from build123d import *

# Parameters (mm, degrees)
T_LE_DE_BASE_PLI_E1_DEPTH             = 20.5
ESQUISSE8_W                           = 24
ESQUISSE8_H                           = 2
BOSS_EXTRU_1_DEPTH                    = 8.5
T_LE_PLI_E_SUR_AR_TE1_STRIP_W         = 10
T_LE_PLI_E_SUR_AR_TE1_STRIP_H         = 2
T_LE_PLI_E_SUR_AR_TE1_STRIP_CUT_DEPTH = 8.5
T_LE_PLI_E_SUR_AR_TE1_DEPTH           = 8.5
ESQUISSE12_W                          = 1.5
ESQUISSE12_H                          = 12
ENL_V_MAT_EXTRU_1_DEPTH               = 8.5
DIAM_TRE_DU_PER_AGE_4_0_4_1_D         = 4
DIAM_TRE_DU_PER_AGE_8_0_8_1_D         = 8
DIAM_TRE_DU_PER_AGE_2_5_2_5_1_D       = 2.5
R_P_TITION_CIRCULAIRE1_COUNT          = 8
DIAM_TRE_DU_PER_AGE_4_0_4_2_D         = 4
DIAM_TRE_DU_PER_AGE_2_5_2_5_2_D       = 2.5
CONG_1_R                              = 4
DIAM_TRE_DU_PER_AGE_8_0_8_2_D         = 8
DIAM_TRE_DU_PER_AGE_2_5_2_5_3_D       = 2.5
R_P_TITION_CIRCULAIRE2_COUNT          = 4
CROQUIS1_R                            = 2.5
CORTAR_EXTRUIR1_DEPTH                 = 10


# Sheet-metal steps are written as plain solids
with BuildPart() as part:
    # Esquisse1 → Tôle de base pliée1 (new body)
    with BuildSketch(Plane(origin=(0, 0, 0), x_dir=(0, 0, -1), z_dir=(1, 0, 0))):
        with BuildLine():
            Line((0, 27), (0, 3))
            ThreePointArc((0, 3), (-0.878679656, 0.878679656), (-3, 0))
            Line((-3, 0), (-37.5, 0))
            Line((-37.5, 0), (-37.5, 2))
            Line((-37.5, 2), (-3, 2))
            ThreePointArc((-3, 2), (-2.292893219, 2.292893219), (-2, 3))
            Line((-2, 3), (-2, 27))
            Line((-2, 27), (0, 27))
        make_face()
    extrude(amount=T_LE_DE_BASE_PLI_E1_DEPTH)

    # Esquisse8 → Boss.-Extru.1 (add)
    with BuildSketch(Plane(origin=(20.5, 0, 0), x_dir=(0, 0, -1), z_dir=(1, 0, 0))):
        with Locations((-19, 1)):
            Rectangle(ESQUISSE8_W, ESQUISSE8_H)
    extrude(amount=BOSS_EXTRU_1_DEPTH)

    # Tôle pliée sur arête1 strip (across the edge) → Tôle pliée sur arête1 strip cut (cut)
    with BuildSketch(Plane(origin=(20.5, 2, 31), x_dir=(0, 0, -1), z_dir=(1, 0, 0))):
        with Locations((-4, -1)):
            Rectangle(T_LE_PLI_E_SUR_AR_TE1_STRIP_W, T_LE_PLI_E_SUR_AR_TE1_STRIP_H)
    extrude(amount=T_LE_PLI_E_SUR_AR_TE1_STRIP_CUT_DEPTH, mode=Mode.SUBTRACT)

    # Tôle pliée sur arête1 section (across the edge) → Tôle pliée sur arête1 (add)
    with BuildSketch(Plane(origin=(20.5, 2, 31), x_dir=(0, 0, -1), z_dir=(1, 0, 0))):
        with BuildLine():
            Line((-2, 1), (-2, 25))
            Line((-2, 25), (0, 25))
            Line((0, 25), (0, 1))
            ThreePointArc((0, 1), (0.292893219, 0.292893219), (1, 0))
            Line((1, 0), (1, -2))
            ThreePointArc((1, -2), (-1.121320344, -1.121320344), (-2, 1))
        make_face()
    extrude(amount=T_LE_PLI_E_SUR_AR_TE1_DEPTH)

    # Esquisse12 → Enlèv. mat.-Extru.1 (cut)
    with BuildSketch(Plane(origin=(0, 2, 0), x_dir=(1, 0, 0), z_dir=(0, 1, 0))):
        with Locations((19.75, -31.5)):
            Rectangle(ESQUISSE12_W, ESQUISSE12_H)
    extrude(amount=-ENL_V_MAT_EXTRU_1_DEPTH, mode=Mode.SUBTRACT)

    # Diamètre du perçage Ø4.0 (4)1 (through all)
    with Locations(Plane(origin=(0, 2, 0), x_dir=(1, 0, 0), z_dir=(0, 1, 0))):
        with Locations((24.25, -12.13), (24.25, -22.13)):
            Hole(DIAM_TRE_DU_PER_AGE_4_0_4_1_D / 2)

    # Diamètre du perçage Ø8.0 (8)1 (through all)
    with Locations(Plane(origin=(0, 2, 0), x_dir=(1, 0, 0), z_dir=(0, 1, 0))):
        with Locations((9.75, -25.5)):
            Hole(DIAM_TRE_DU_PER_AGE_8_0_8_1_D / 2)

    # Diamètre du perçage Ø2.5 (2.5)1 (through all)
    with Locations(Plane(origin=(0, 2, 0), x_dir=(1, 0, 0), z_dir=(0, 1, 0))):
        with Locations((9.75, -18.5)):
            diam_tre_du_per_age_2_5_2_5_1 = Hole(DIAM_TRE_DU_PER_AGE_2_5_2_5_1_D / 2)

    # Répétition circulaire1: Diamètre du perçage Ø2.5 (2.5)1 ×8 about axis, 3 skipped
    r_p_tition_circulaire1_axis = Axis((9.75, 2, 25.5), (0, 1, 0))
    add([diam_tre_du_per_age_2_5_2_5_1.rotate(r_p_tition_circulaire1_axis, i * 360 / R_P_TITION_CIRCULAIRE1_COUNT) for i in range(1, R_P_TITION_CIRCULAIRE1_COUNT) if i not in (1, 3, 6)], mode=Mode.SUBTRACT)

    # Diamètre du perçage Ø4.0 (4)2 (through all)
    with Locations(Plane.XY.offset(33)):
        with Locations((24.25, 19.87), (24.25, 9.87)):
            Hole(DIAM_TRE_DU_PER_AGE_4_0_4_2_D / 2)

    # Diamètre du perçage Ø2.5 (2.5)2 (through all)
    with Locations(Plane.XY.offset(2)):
        with Locations((10, 14.87)):
            Hole(DIAM_TRE_DU_PER_AGE_2_5_2_5_2_D / 2)

    # Congé1
    cong_1_edges = [part.edges().sort_by_distance(p)[0] for p in [
        (20.5, 27, 1),
        (29, 1, 7),
        (29, 27, 32),
        (19, 1, 37.5),
    ]]
    fillet(cong_1_edges, radius=CONG_1_R)

    # Symétrie1: part across plane


with BuildPart() as part_1:
    add(part.part)
    add(part.part.mirror(Plane(origin=(0, 3, 3), x_dir=(0, 0, 1), z_dir=(1, 0, 0))))

    # Diamètre du perçage Ø8.0 (8)2 (through all)
    with Locations(Plane(origin=(0, 2, 0), x_dir=(1, 0, 0), z_dir=(0, 1, 0))):
        with Locations((0, -12.13)):
            Hole(DIAM_TRE_DU_PER_AGE_8_0_8_2_D / 2)

    # Diamètre du perçage Ø2.5 (2.5)3 (through all)
    with Locations(Plane(origin=(0, 2, 0), x_dir=(1, 0, 0), z_dir=(0, 1, 0))):
        with Locations((0, -5.13)):
            diam_tre_du_per_age_2_5_2_5_3 = Hole(DIAM_TRE_DU_PER_AGE_2_5_2_5_3_D / 2)

    # Répétition circulaire2: Diamètre du perçage Ø2.5 (2.5)3 ×4 about axis
    r_p_tition_circulaire2_axis = Axis((0, 0, 12.13), (0, 1, 0))
    for i in range(1, R_P_TITION_CIRCULAIRE2_COUNT):
        add(diam_tre_du_per_age_2_5_2_5_3.rotate(r_p_tition_circulaire2_axis, i * 360 / R_P_TITION_CIRCULAIRE2_COUNT), mode=Mode.SUBTRACT)

    # Croquis1 → Cortar-Extruir1 (cut)
    with BuildSketch(Plane.XY.offset(2)):
        with Locations((10, 14.87)):
            Circle(CROQUIS1_R)
        with Locations((-10, 14.87)):
            Circle(CROQUIS1_R)
    extrude(amount=-CORTAR_EXTRUIR1_DEPTH, mode=Mode.SUBTRACT)


solid = part_1.part
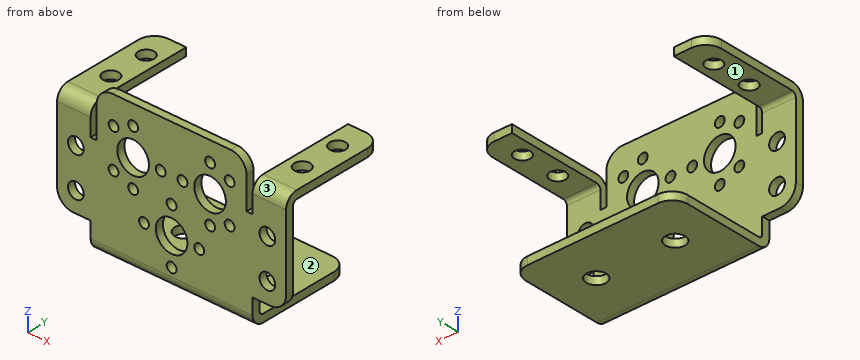
For this review, take the finished solid that the model builds, in its own axes (mm). Face numbers are marked on the shaded views. A direction names the side the tool comes from. Round coordinates to 2 decimals unless told otherwise and drop trailing zeros. Write each loop counter-clockwise with the first axis right and the second up, starting at its lowest first coordinate (ties: lowest second). Pieces come first, ordered by that corner, then holes. Notation, with made-up numbers: (25.25, 11) - (58.25, 11) arc R12 cw to (58.25, 31) - close; hole circle Ø10 at (19, -9.75). An arc over 180 degrees is marked (long way). Use a Markdown table: item, result.
Q1. We need section B-B (y = 14.87). Give the boundary of the cut face in (x, z), plus the area to 3 significant figures.
Derived:
| item | result |
|---|---|
| outline | (-29, 31) - (-20.5, 31) - (-20.5, 33) - (-29, 33) - close; (-20.5, 0) - (-12.5, 0) - (-12.5, 2) - (-20.5, 2) - close; (-7.5, 0) - (7.5, 0) - (7.5, 2) - (-7.5, 2) - close; (12.5, 0) - (20.5, 0) - (20.5, 2) - (12.5, 2) - close; (20.5, 31) - (29, 31) - (29, 33) - (20.5, 33) - close |
| area | 96.0 mm2 |
Q2. We need section D-D (x = -10). Give the boundary of the cut face in (y, z), plus the area to 3 significant figures.
Derived:
| item | result |
|---|---|
| outline | (0, 3) arc R3 ccw to (3, 0) - (12.37, 0) - (12.37, 2) - (3, 2) arc R1 cw to (2, 3) - (2, 17.28) - (0, 17.28) - close; (0, 19.72) - (2, 19.72) - (2, 21.51) - (0, 21.51) - close; (0, 29.49) - (2, 29.49) - (2, 31.28) - (0, 31.28) - close; (0, 33.72) - (2, 33.72) - (2, 37.5) - (0, 37.5) - close; (17.37, 0) - (27, 0) - (27, 2) - (17.37, 2) - close |
| area | 87.5 mm2 |
Q3. Wall thickness on line 1 along X through (y, z) = (0.8, 22.13); line 2 along Z through (x, y) = (-9.75, 1.1); line 3 along X through (y, z) = (1.3, 18.5): over which ranges is each line inside the solid? List them lowest first.
Derived:
| item | result |
|---|---|
| line 1 | x = -29 to -26.25, -22.25 to -11.9, -7.6 to 7.6, 11.9 to 22.25, 26.25 to 29 |
| line 2 | z = 0.68 to 17.25, 19.75 to 21.5, 29.5 to 31.25, 33.75 to 37.5 |
| line 3 | x = -29 to -11, -8.5 to -1.08, 1.08 to 8.5, 11 to 29 |
Q4. Machinability: for the marked faces 1, 2 and 3, which of the approach directions +Z, -Z, +X, -X, +Y, -Y give a long, thin tool a straight path to every point of the face, cutting with its end or side? Answer none if there is none.
Derived:
| item | result |
|---|---|
| face 1 | -Z, +X, -X, +Y |
| face 2 | +Z, +X, -X, +Y |
| face 3 | +Z, +X, -Y |
Q5. We need section A-A (x = 0). Give the boundary of the cut face in (y, z), plus the area to 3 significant figures.
Derived:
| item | result |
|---|---|
| outline | (0, 3) arc R3 ccw to (3, 0) - (27, 0) - (27, 2) - (3, 2) arc R1 cw to (2, 3) - (2, 3.88) - (0, 3.88) - close; (0, 6.38) - (2, 6.38) - (2, 8.13) - (0, 8.13) - close; (0, 16.13) - (2, 16.13) - (2, 17.88) - (0, 17.88) - close; (0, 20.38) - (2, 20.38) - (2, 37.5) - (0, 37.5) - close |
| area | 97.3 mm2 |
Q6. We need section C-C (z = 12.13). Give the boundary of the cut face in (x, y), plus the area to 3 significant figures.
Derived:
| item | result |
|---|---|
| outline | (-29, 0) - (-26.25, 0) - (-26.25, 2) - (-29, 2) - close; (-22.25, 0) - (-8.25, 0) - (-8.25, 2) - (-22.25, 2) - close; (-5.75, 0) - (-4, 0) - (-4, 2) - (-5.75, 2) - close; (4, 0) - (5.75, 0) - (5.75, 2) - (4, 2) - close; (8.25, 0) - (22.25, 0) - (22.25, 2) - (8.25, 2) - close; (26.25, 0) - (29, 0) - (29, 2) - (26.25, 2) - close |
| area | 74.0 mm2 |
Q7. Clearance check with flat-ended pins moving along their axes: pin 1 (3 mm diameter, centred on x = -24.25, y = 19.87, fed in from -Z); pin 2 (3 mm diameter, centred on x = -14.7, z = 30.45, fed in from +Y); pin 3 (8 mm diameter, centred on x = -5.5, y = 21.5, fed in from +Z); pin 4 (7 mm diameter, centred on x = -26.5, y = 14.5, fed in from +Z). State where each tip first meets the part, or that it passes through.
Derived:
| item | result |
|---|---|
| pin 1 | passes through |
| pin 2 | stops at y = 2 |
| pin 3 | stops at z = 2 |
| pin 4 | stops at z = 33 |
